from build123d import *

# Parameters (mm, degrees)
F1_DEPTH = 1.4
F2_W     = 0.5
F2_H     = 21
F3_DEPTH = 3.7
F5_D     = 3.5
F7_DEPTH = 0.25
F8_R     = 0.24999
F9_R     = 0.4999


# Not quite as in the source:
# - a fillet or chamfer is up to 0.001 mm smaller than in the source, because OpenCascade refuses the exact size


with BuildPart() as f1:
    # F0 (on Right) → F1 (new body)
    with BuildSketch(Plane.YZ):
        Polygon((0, 9.2), (0, 0), (23.5, 0), (23.5, 13), (2.5, 13), (2.5, 9.2), align=None)
    extrude(amount=F1_DEPTH)

    # F2 (on face) → F3 (join)
    with BuildSketch(Plane.XY.offset(13)):
        with Locations((0.25, 13)):
            Rectangle(F2_W, F2_H)
    extrude(amount=F3_DEPTH)

    # F5 (through all)
    with Locations(Plane.YZ.offset(1.4)):
        with Locations((6, 3.1), (15, 3.1)):
            Hole(F5_D / 2)

    # F6 (on face) → F7 (join)
    with BuildSketch(Plane.YZ.offset(0.5)):
        with BuildLine():
            Line((7.9, 16.7), (7.9, 14))
            ThreePointArc((7.9, 14), (7.6071067812, 13.2928932188), (6.9, 13))
            Line((6.9, 13), (7.9, 13))
            Line((7.9, 13), (8.15, 13))
            Line((8.15, 13), (9.15, 13))
            ThreePointArc((9.15, 13), (8.4428932188, 13.2928932188), (8.15, 14))
            Line((8.15, 14), (8.15, 16.7))
            Line((8.15, 16.7), (7.9, 16.7))
        make_face()
        with BuildLine():
            Line((18.1, 16.7), (17.85, 16.7))
            Line((17.85, 16.7), (17.85, 14))
            ThreePointArc((17.85, 14), (17.5571067812, 13.2928932188), (16.85, 13))
            Line((16.85, 13), (17.85, 13))
            Line((17.85, 13), (18.1, 13))
            Line((18.1, 13), (19.1, 13))
            ThreePointArc((19.1, 13), (18.3928932188, 13.2928932188), (18.1, 14))
            Line((18.1, 14), (18.1, 16.7))
        make_face()
    extrude(amount=F7_DEPTH)

    # F8 (radius 0.25 in the source; OpenCascade refuses exactly that, so slightly less here)
    f8_edges = [f1.edges().sort_by_distance(p)[0] for p in [
        (0, 13, 16.7),
        (0.5, 20.8, 16.7),
        (0.5, 13, 16.7),
        (0.5, 5.2, 16.7),
    ]]
    fillet(f8_edges, radius=F8_R)

    # F9 (radius 0.5 in the source; OpenCascade refuses exactly that, so slightly less here)
    f9_edges = [f1.edges().sort_by_distance(p)[0] for p in [
        (0.75, 8.025, 16.7),
        (0.75, 17.975, 16.7),
    ]]
    fillet(f9_edges, radius=F9_R)


solid = f1.part
Check sheet for the modelled part. Datum: model origin and axes. Units: mm. A direction names the side the tool comes from. Round coordinates to 2 decimals unless told otherwise and drop trailing zeros. Loops run counter-clockwise (first coordinate to the right, second up) from the corner with the lowest first, then second, coordinate; pieces in that order, holes last. Notation, with made-up numbers: (28, 6) -> (42, 6) arc R24 ccw to (42, 31) -> close; hole circle Ø10 at (68, -28.5). An arc over 180 degrees is marked (long way). Put each result on its own line as item: value. Start each with the question number.
1. Scan lines: probe 1 along Z at (x, y) = (0.95, 15); probe 2 along Y at (x, z) = (0.6, 12); probe 3 along Z at (x, y) = (0.25, 4.5). Record each from-to range of solid material in increasing order.
2. Draft check along Z on faces 4 (the face through (1, 12, 0)), 5 (the face through (0.69, 7.75, 3.18)), 6 (the face through (1, 2.5, 12)), 7 (the face through (0.69, 13.331, 3.626)). Enter one of: +Z half, -Z half, draft (parallel to the pull), parting line (faces both ways), or undercut.
3. Gauge pin test, flat ends, axial feed: pin 1 (3 mm diameter, centred on y = 4, z = 15, fed in from +X); pin 2 (1.1 mm diameter, centred on y = 18.5, z = 14.5, fed in from +X); pin 3 (0.7 mm diameter, centred on x = 1, y = 10, fed in from +Z). Record the tip position at first contact, or that the pin passes through.
4. Section check A-A (z = 3.1). Enter the section's corners in (x, y), plus the area to 3 significant figures.
5. Section check C-C (x = 1.1). Enter the section's corners in (y, z).
6. Access from +Z, -Z, +X, -X, +Y, -Y to the whole of each face (thin tool, end or side, straight path). Record for faces 1 (the face through (0.5, 21, 15)), 2 (the face through (0.5, 13, 15)), 3 (the face through (1, 1, 9.2)).
Findings:
1. probe 1: z = 0 to 1.35, 4.85 to 13
1. probe 2: y = 2.5 to 23.5
1. probe 3: z = 0 to 2.2, 4 to 16.7
2. face 4: -Z half
2. face 5: undercut
2. face 6: draft
2. face 7: undercut
3. pin 1: stops at x = 0.5
3. pin 2: stops at x = 0.75
3. pin 3: stops at z = 13
4. outline: (0, 0) -> (1.4, 0) -> (1.4, 4.25) -> (0, 4.25) -> close; (0, 7.75) -> (1.4, 7.75) -> (1.4, 13.25) -> (0, 13.25) -> close; (0, 16.75) -> (1.4, 16.75) -> (1.4, 23.5) -> (0, 23.5) -> close
4. area: 23.1 mm^2
5. outline: (0, 0) -> (23.5, 0) -> (23.5, 13) -> (2.5, 13) -> (2.5, 9.2) -> (0, 9.2) -> close; hole circle Ø3.5 at (6, 3.1); hole circle Ø3.5 at (15, 3.1)
6. face 1: +Z, +X, +Y
6. face 2: +Z, +X
6. face 3: +Z, +X, -X, -Y
